from build123d import *

# Parameters (mm, degrees)
SKETCH1_W           = 138.1125
SKETCH1_H           = 39.6875
SKETCH1_W_2         = 131.7625
SKETCH1_H_2         = 33.3375
BOSS_EXTRUDE1_DEPTH = 14.2875
SKETCH2_W           = 138.1125
SKETCH2_H           = 39.6875
BOSS_EXTRUDE2_DEPTH = 3.175
CUT_EXTRUDE1_REACH  = 142.26
SKETCH3_W           = 14.2875
SKETCH3_H           = 33.3375
BOSS_EXTRUDE3_REACH = 142.26
SKETCH4_W           = 2.38125
SKETCH4_H           = 2.38125
BOSS_EXTRUDE4_START = -8.73125
SKETCH6_W           = 138.1125
SKETCH6_H           = 12.7
SKETCH6_R           = 2.5
BOSS_EXTRUDE4_DEPTH = 1.5
SKETCH7_R           = 2.95
CUT_EXTRUDE2_DEPTH  = 1
SKETCH8_W           = 9.525
SKETCH8_H           = 9.525
BOSS_EXTRUDE5_DEPTH = 9.525
BOSS_EXTRUDE6_START = -10.23125
SKETCH9_W           = 15.875
SKETCH9_H           = 12.7
SKETCH9_R           = 3.175
BOSS_EXTRUDE6_DEPTH = 7.23125


with BuildPart() as part:
    # Sketch1 → Boss-Extrude1 (new body)
    with BuildSketch(Plane.XY):
        Rectangle(SKETCH1_W, SKETCH1_H)
        Rectangle(SKETCH1_W_2, SKETCH1_H_2, mode=Mode.SUBTRACT)
    extrude(amount=BOSS_EXTRUDE1_DEPTH)

    # Sketch2 → Boss-Extrude2 (add)
    with BuildSketch(Plane(origin=(0, 0, 0), x_dir=(-1, 0, 0), z_dir=(0, 0, -1))):
        Rectangle(SKETCH2_W, SKETCH2_H)
    extrude(amount=BOSS_EXTRUDE2_DEPTH)

    # Sketch3 → Cut-Extrude1 (cut, up to next)
    with BuildSketch(Plane(origin=(69.05625, 0, 0), x_dir=(0, 0, -1), z_dir=(1, 0, 0)), mode=Mode.PRIVATE) as cut_extrude1_sk1:
        with Locations((-7.14375, 0)):
            Rectangle(SKETCH3_W, SKETCH3_H)
    cut_extrude1_tool1 = extrude(cut_extrude1_sk1.sketch, amount=-CUT_EXTRUDE1_REACH, mode=Mode.PRIVATE) & part.part
    add(cut_extrude1_tool1.solids().sort_by_distance((69.05625, 0, 7.14375))[0], mode=Mode.SUBTRACT)

    # Sketch4 → Boss-Extrude3 (add, up to next)
    with BuildSketch(Plane(origin=(69.05625, 0, 0), x_dir=(0, 0, -1), z_dir=(1, 0, 0)), mode=Mode.PRIVATE) as boss_extrude3_sk1:
        with Locations((-5.953125, -15.478125)):
            Rectangle(SKETCH4_W, SKETCH4_H)
    boss_extrude3_tool1 = extrude(boss_extrude3_sk1.sketch, amount=-BOSS_EXTRUDE3_REACH, mode=Mode.PRIVATE) - part.part
    # Sketch4 → Boss-Extrude3 (add, up to next)
    with BuildSketch(Plane(origin=(69.05625, 0, 0), x_dir=(0, 0, -1), z_dir=(1, 0, 0)), mode=Mode.PRIVATE) as boss_extrude3_sk2:
        with Locations((-5.953125, 15.478125)):
            Rectangle(SKETCH4_W, SKETCH4_H)
    boss_extrude3_tool2 = extrude(boss_extrude3_sk2.sketch, amount=-BOSS_EXTRUDE3_REACH, mode=Mode.PRIVATE) - part.part
    add(boss_extrude3_tool1.solids().sort_by_distance((69.05625, -15.478125, 5.953125))[0])
    add(boss_extrude3_tool2.solids().sort_by_distance((69.05625, 15.478125, 5.953125))[0])

    # Sketch6 → Boss-Extrude4 (add, symmetric)
    with BuildSketch(Plane(origin=(0, 0, -3.175), x_dir=(-1, 0, 0), z_dir=(0, 0, -1)).offset(BOSS_EXTRUDE4_START)):
        with Locations((0, 26.19375)):
            Rectangle(SKETCH6_W, SKETCH6_H)
        with Locations((0, 26.19375)):
            Circle(SKETCH6_R, mode=Mode.SUBTRACT)
        with Locations((-53.18125, 26.19375)):
            Circle(SKETCH6_R, mode=Mode.SUBTRACT)
        with Locations((53.18125, 26.19375)):
            Circle(SKETCH6_R, mode=Mode.SUBTRACT)
    extrude(amount=BOSS_EXTRUDE4_DEPTH, both=True)

    # Sketch7 → Cut-Extrude2 (cut)
    with BuildSketch(Plane(origin=(0, 0, 4.05625), x_dir=(-1, 0, 0), z_dir=(0, 0, -1))):
        with Locations((-53.18125, 26.19375)):
            Circle(SKETCH7_R)
        with Locations((0, 26.19375)):
            Circle(SKETCH7_R)
        with Locations((53.18125, 26.19375)):
            Circle(SKETCH7_R)
    extrude(amount=-CUT_EXTRUDE2_DEPTH, mode=Mode.SUBTRACT)

    # Sketch8 → Boss-Extrude5 (add)
    with BuildSketch(Plane.XZ.offset(19.84375)):
        with Locations((0, 1.5875)):
            Rectangle(SKETCH8_W, SKETCH8_H)
    extrude(amount=BOSS_EXTRUDE5_DEPTH)

    # Sketch9 → Boss-Extrude6 (add)
    # profile 1 of 4: a face of its own
    with BuildSketch(Plane.XY.offset(7.05625).offset(BOSS_EXTRUDE6_START)):
        with Locations((-34.925, 26.19375)):
            Rectangle(SKETCH9_W, SKETCH9_H)
    # profile 2 of 4: a face of its own
    with BuildSketch(Plane.XY.offset(7.05625).offset(BOSS_EXTRUDE6_START)):
        with BuildLine():
            Line((-42.8625, 45.24375), (-42.8625, 32.54375))
            Line((-42.8625, 32.54375), (-26.9875, 32.54375))
            Line((-26.9875, 32.54375), (-26.9875, 45.24375))
            ThreePointArc((-26.9875, 45.24375), (-34.925, 53.18125), (-42.8625, 45.24375))
        make_face()
        with Locations(Location((-34.925, 45.24375, 0), (0, 0, 180))):
            Circle(SKETCH9_R, mode=Mode.SUBTRACT)
    # profile 3 of 4: a face of its own
    with BuildSketch(Plane.XY.offset(7.05625).offset(BOSS_EXTRUDE6_START)):
        with Locations((34.925, 26.19375)):
            Rectangle(SKETCH9_W, SKETCH9_H)
    # profile 4 of 4: a face of its own
    with BuildSketch(Plane.XY.offset(7.05625).offset(BOSS_EXTRUDE6_START)):
        with BuildLine():
            Line((26.9875, 45.24375), (26.9875, 32.54375))
            Line((26.9875, 32.54375), (42.8625, 32.54375))
            Line((42.8625, 32.54375), (42.8625, 45.24375))
            ThreePointArc((42.8625, 45.24375), (34.925, 53.18125), (26.9875, 45.24375))
        make_face()
        with Locations(Location((34.925, 45.24375, 0), (0, 0, 180))):
            Circle(SKETCH9_R, mode=Mode.SUBTRACT)
    extrude(amount=BOSS_EXTRUDE6_DEPTH)


solid = part.part
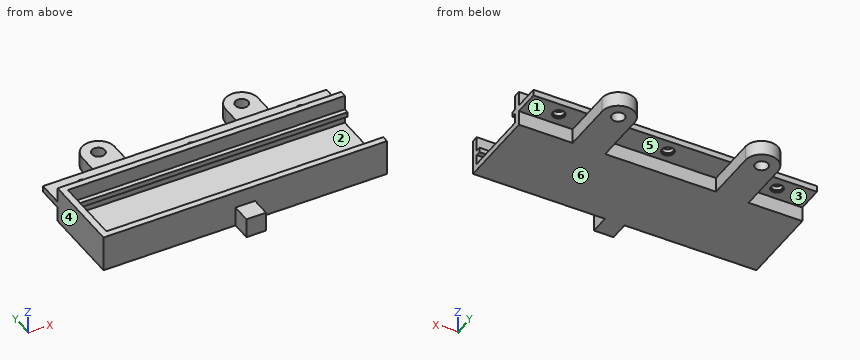
Geometry: final body of the model. Coordinates: model frame, mm. Face numbers are marked on the shaded views. A direction names the side the tool comes from. Coordinates: 2 decimals unless noted, no trailing zeros. Loops run counter-clockwise (first coordinate to the right, second up) from the corner with the lowest first, then second, coordinate; pieces in that order, holes last. Notation, with made-up numbers: (52, 46) - (83, 46) arc R28 ccw to (83, 72) - close; hole circle Ø4 at (79.5, 46). An arc over 180 degrees is marked (long way). Put each result on its own line as item: value. Start each with the question number.
Q1. Line query: line 1 (Y direction, x = 0, z = 4.4); line 2 (Y direction, x = -8, z = 12.75); line 3 (Y direction, x = 15, z = 5). Output: solid intervals per line, ascending.
Q2. Pin query (flat end, axial travel): pin 1 Ø6 at (y, z) = (36.5, 2) entering from +X; pin 2 Ø3.5 at (y, z) = (30.5, 1) entering from -X; pin 3 Ø8 at (x, y) = (-48, 27) entering from +Z. Return the tip coordinate at first contact, or that it passes through.
Q3. Cut plane C-C, the plane y = 43.5. Return loops of the section in (x, z) (1 decimal).
Q4. Cut plane B-B, the plane x = -23.5. Return loops of the section in (y, z) (1 decimal).
Q5. Cut plane D-D, the plane y = 4. Return loops of the section in (x, z) (1 decimal).
Q6. Pull-direction query (X, two-part tool) for the marked faces 4, 5 and 6; classes: released by +X, released by -X, zero draft, split by the parting line, or undercut.
Q7. Set-up query: the marked faces 1, 2 and 3. Return all of +Z, -Z, +X, -X, +Y, -Y with unobstructed straight access to the full face (end or side cutting, diameter ignored); none if empty.
Filled sheet:
1. line 1: -29.37 to -16.67, 16.67 to 23.24, 29.14 to 32.54
1. line 2: -19.84 to -16.67, 16.67 to 19.84
1. line 3: -19.84 to -14.29, 14.29 to 32.54
2. pin 1: x = 42.86
2. pin 2: x = -42.86
2. pin 3: z = 7.06
3. outline: (-42.9, -3.2) - (-37.6, -3.2) - (-37.6, 4.1) - (-42.9, 4.1) - close; (-32.3, -3.2) - (-27, -3.2) - (-27, 4.1) - (-32.3, 4.1) - close; (27, -3.2) - (32.3, -3.2) - (32.3, 4.1) - (27, 4.1) - close; (37.6, -3.2) - (42.9, -3.2) - (42.9, 4.1) - (37.6, 4.1) - close
4. outline: (-19.8, -3.2) - (19.8, -3.2) - (19.8, 4.1) - (32.5, 4.1) - (32.5, 7.1) - (19.8, 7.1) - (19.8, 14.3) - (16.7, 14.3) - (16.7, 7.1) - (14.3, 7.1) - (14.3, 4.8) - (16.7, 4.8) - (16.7, 0) - (-16.7, 0) - (-16.7, 4.8) - (-14.3, 4.8) - (-14.3, 7.1) - (-16.7, 7.1) - (-16.7, 14.3) - (-19.8, 14.3) - close
5. outline: (-69.1, -3.2) - (69.1, -3.2) - (69.1, 0) - (-65.9, 0) - (-65.9, 14.3) - (-69.1, 14.3) - close
6. face 4: released by -X
6. face 5: undercut
6. face 6: zero draft
7. face 1: -Z, +X, +Y
7. face 2: +X
7. face 3: -Z, -X, +Y
